Work out the finished part from the listing and answer in its coordinate system (mm). A direction names the side the tool comes from. Round coordinates to 2 decimals unless told otherwise and drop trailing zeros. Loops run counter-clockwise (first coordinate to the right, second up) from the corner with the lowest first, then second, coordinate; pieces in that order, holes last. Notation, with made-up numbers: (34, -2.75) - (58, -2.75) arc R23 ccw to (58, 17.25) - close; hole circle Ø11 at (-25.5, 63.5). An arc over 180 degrees is marked (long way). Use CSV: the item, a comma, the result in double quotes. Start each with the question number.
from build123d import *

# Parameters (mm, degrees)
SKETCH_1_W          = 49.901037986
SKETCH_1_H          = 11.5
EXTRUDE_1_DEPTH     = 3
SKETCH_3_W          = 11.5
SKETCH_3_H          = 23
EXTRUDE_2_DEPTH     = 2
SKETCH_4_R          = 4
CUT_EXTRUDE_1_DEPTH = 3
SKETCH_7_W          = 44.527674248
SKETCH_7_H          = 38.163809885
CUT_EXTRUDE_2_DEPTH = 10
EXTRUDE_3_DEPTH     = 11.5
SKETCH_9_R          = 1.1
CUT_EXTRUDE_3_DEPTH = 10
FILLET_2_R          = 3
FILLET_3_R          = 3


with BuildPart() as part:
    # 草图1 → 凸台-拉伸1 (new body)
    with BuildSketch(Plane(origin=(0, 0, 0), x_dir=(1, 0, 0), z_dir=(0, 1, 0))):
        Rectangle(SKETCH_1_W, SKETCH_1_H)
    extrude(amount=EXTRUDE_1_DEPTH)

    # 草图3 → 凸台-拉伸2 (add)
    with BuildSketch(Plane.ZY.offset(24.950518993)):
        with Locations((0, 11.5)):
            Rectangle(SKETCH_3_W, SKETCH_3_H)
    extrude(amount=-EXTRUDE_2_DEPTH)

    # 草图4 → 切除-拉伸1 (cut)
    with BuildSketch(Plane(origin=(-22.950518993, 0, 0), x_dir=(0, 0, -1), z_dir=(1, 0, 0))):
        with Locations((0, 17.25)):
            Circle(SKETCH_4_R)
    extrude(amount=-CUT_EXTRUDE_1_DEPTH, mode=Mode.SUBTRACT)

    # 草图7 → 切除-拉伸2 (cut)
    with BuildSketch(Plane(origin=(0, 3, 0), x_dir=(1, 0, 0), z_dir=(0, 1, 0))):
        with Locations((10.77056276, -2.40663606)):
            Rectangle(SKETCH_7_W, SKETCH_7_H)
    extrude(amount=-CUT_EXTRUDE_2_DEPTH, mode=Mode.SUBTRACT)

    # 草图8 → 凸台-拉伸3 (add)
    with BuildSketch(Plane.XY.offset(5.75)):
        Polygon((-22.950518993, 9.295590995), (-22.950518993, 3), (-20.10387752, 3), align=None)
    extrude(amount=-EXTRUDE_3_DEPTH)

    # 草图9 → 切除-拉伸3 (cut)
    with BuildSketch(Plane(origin=(0, 3, 0), x_dir=(1, 0, 0), z_dir=(0, 1, 0))):
        with Locations(Location((-15.798575942, 3, 0), (0, 0, 270))):
            Circle(SKETCH_9_R)
        with Locations(Location((-15.798575942, -3, 0), (0, 0, 270))):
            Circle(SKETCH_9_R)
    extrude(amount=-CUT_EXTRUDE_3_DEPTH, mode=Mode.SUBTRACT)

    # 圆角2
    fillet_2_edges = [part.edges().sort_by_distance(p)[0] for p in [
        (-23.950518993, 23, -5.75),
        (-23.950518993, 23, 5.75),
    ]]
    fillet(fillet_2_edges, radius=FILLET_2_R)

    # 圆角3
    fillet_3_edges = [part.edges().sort_by_distance(p)[0] for p in [
        (-11.493274364, 1.5, 5.75),
        (-11.493274364, 1.5, -5.75),
    ]]
    fillet(fillet_3_edges, radius=FILLET_3_R)


solid = part.part
Item 1: Which of the six approach directions +Z, -Z, +X, -X, +Y, -Y give full straight-line access (tool end or side, diameter ignored) to faces 4 (the flat face through (-22.951, 13, 0)), 5 (the flat face through (-22, 6, -5.75))?
Item 2: A cutting plane is placed at C-C (x = -23.25). Determine the outline of the cut face in (y, z), plus the area to 3 significant figures.
Item 3: A cutting plane is placed at B-B (z = 0). Determine the outline of the cut face in (x, y).
Item 4: A cutting plane is placed at A-A (y = 17.25). Determine the outline of the cut face in (x, z), plus the area to 3 significant figures.
Item 5: Each of these flat-tipped pins is pushed along its axis until it touches: pin 1 Ø3 at (x, z) = (-15.8, -3) entering from +Y; pin 2 Ø5 at (y, z) = (5, 2.5) entering from +X; pin 3 Ø3.5 at (y, z) = (17, 2.5) entering from +X. Where does it stop, or does it pass through?
Item 6: A cutting plane is placed at D-D (z = -3). Determine the outline of the cut face in (x, y).
Item 7: Find the intervals of material crossed by probe 1 along Y at (x, z) = (-23.85, 0); probe 2 along X at (y, z) = (19.5, 4.25); probe 3 along Y at (x, z) = (-23, 1.75), in increasing order. Write a range as [from, to].
Item 8: The mould has two halves that part along Y. Classify faces 1 (the flat face through (-24.951, 11, 0)), 2 (the flat face through (-24, 23, 0)), 3 (the cylindrical face through (-23.937, 21.216, 0.521)): pulls with the +Y half, pulls with the -Y half, needs draft (parallel to the pull), parting line crosses it, or undercut.
Result sheet:
1,face 4,"+Z, -Z, +X, +Y"
1,face 5,"-Z, +X, -X, +Y, -Y"
2,outline,"(0, -5.75) - (20, -5.75) arc R3 ccw to (23, -2.75) - (23, 2.75) arc R3 ccw to (20, 5.75) - (0, 5.75) - close; hole circle Ø8 at (17.25, 0)"
2,area,"210 mm^2"
3,outline,"(-24.95, 0) - (-11.49, 0) - (-11.49, 3) - (-20.1, 3) - (-22.95, 9.3) - (-22.95, 13.25) - (-24.95, 13.25) - close; (-24.95, 21.25) - (-22.95, 21.25) - (-22.95, 23) - (-24.95, 23) - close"
4,outline,"(-24.95, -5.75) - (-22.95, -5.75) - (-22.95, -4) - (-24.95, -4) - close; (-24.95, 4) - (-22.95, 4) - (-22.95, 5.75) - (-24.95, 5.75) - close"
4,area,"7.00 mm^2"
5,pin 1,"y = 3"
5,pin 2,"x = -11.49"
5,pin 3,"x = -22.95"
6,outline,"(-24.95, 0) - (-16.9, 0) - (-16.9, 3) - (-20.1, 3) - (-22.95, 9.3) - (-22.95, 14.6) - (-24.95, 14.6) - close; (-24.95, 19.9) - (-22.95, 19.9) - (-22.95, 22.99) - (-24.95, 22.99) - close; (-14.7, 0) - (-11.5, 0) - (-11.5, 3) - (-14.7, 3) - close"
7,probe 1,"[0, 13.25], [21.25, 23]"
7,probe 2,"[-24.95, -22.95]"
7,probe 3,"[0, 13.65], [20.85, 23]"
8,face 1,"needs draft"
8,face 2,"pulls with the +Y half"
8,face 3,"undercut"
